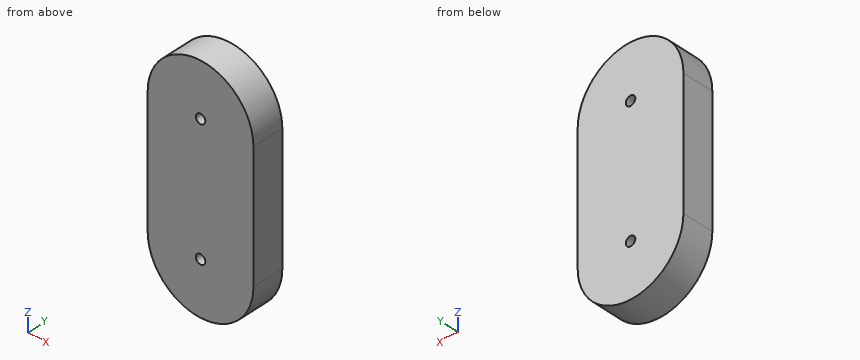
Autodesk Inventor part; units mm, degrees
ref_plane "YZ Plane" through (0, 0, 0) normal (1, 0, 0) x (0, 1, 0)
ref_plane "XZ Plane" through (0, 0, 0) normal (0, 1, 0) x (-1, 0, 0)
ref_plane "XY Plane" through (0, 0, 0) normal (0, 0, 1) x (1, 0, 0)
sketch "Sketch1" plane through (0, 0, 0) normal (0, 1, 0) x (-1, 0, 0)
  line L0 (0, 0) -> (-5.6352, 0)
  line L1 (-5.6352, 0) -> (0, 0)
  line L2 (0, 0) -> (0, 8.7024)
  line L3 (6.5, 14) -> (-6.5, 14)
  line L4 (-6.5, 14) -> (-6.5, 0)
  line L5 (-6.5, 0) -> (6.5, 0)
  line L6 (6.5, 0) -> (6.5, 14)
  circle A0 centre (0, -5) radius 0.9
  circle A1 centre (0, 19) radius 0.9
  line L7 (0, 19) -> (0, -5)
  line L8 (0, 19) -> (0, -5) construction
  line L9 (-10, 19) -> (-10, -5)
  line L10 (10, -5) -> (10, 19)
  arc A2 (10, 19) -> (-10, 19) centre (0, 19) ccw
  arc A3 (-10, -5) -> (10, -5) centre (0, -5) ccw
  point P0 (0, -8.7024)
  point P1 (0, 7)
  dimension "d25" = 13
  dimension "d26" = 14
  dimension "d30" = 5
  dimension "d31" = 5
  dimension "d32" = 1.8
  dimension "d33" = 20
extrude "Extrusion1" add sketch "Sketch1" along normal blind 6 contours L0 L5 L4 L3 L7 L2 | L2 L7 L3 L6 L5 | A2 L10 A3 L9
properties part number "case_usb_cap" material "Acrylic, Clear"
Design review of the part built by this model. Coordinates are the model's own, in mm. Give positions to 0.01 mm unless a question says otherwise; leave off trailing zeros. Order: outer loops, then holes, each group sorted by start corner. A loop starts at its lowest first (then second) coordinate and runs counter-clockwise, first axis right, second up. Notation, with made-up numbers: (51.5, -13) - (74.5, -13) arc R21 ccw to (74.5, -9) - close; hole circle Ø9 at (44.25, 24). An arc over 180 degrees is marked (long way). Use CSV: the item, a comma, the result in double quotes. Start each with the question number.
Q1. Take a section at B-B (y = 0.9). State the section outline as (x, z) points, and give its area (3 significant figures).
Q2. Take a section at D-D (x = -7.5). State the section outline as (y, z) points.
Q3. For P1, Ø3, axis at x = -6, y = 2, coming from the +Z side; P2, Ø1.6, axis at x = 0, z = -5, coming from the -Y side; P3, Ø1.5, axis at x = -3, y = 0.5, coming from the -Z side, all flat-tipped, find the tip position at first contact; note any pin that passes through.
Q4. For line 1 (Z direction, x = 0, y = 3.1); line 2 (X direction, y = 2.7, z = -5); line 3 (Z direction, x = -1.25, y = 0.9), list the stretches that pass through material, from the lowest coordinate up.
Q5. Take a section at C-C (z = -10.5). State the section outline as (x, y) points, and give its area (3 significant figures).
Q6. Take a section at A-A (x = 0). State the section outline as (y, z) points.
Calculated:
1,outline,"(-10, -5) arc R10 ccw to (10, -5) - (10, 19) arc R10 ccw to (-10, 19) - close; hole circle Ø1.8 at (0, -5); hole circle Ø1.8 at (0, 19)"
1,area,"789 mm²"
2,outline,"(0, -11.61) - (6, -11.61) - (6, 25.61) - (0, 25.61) - close"
3,P1,"stops at z = 27.93"
3,P2,"passes through"
3,P3,"stops at z = -14.74"
4,line 1,"z = -15 to -5.9, -4.1 to 18.1, 19.9 to 29"
4,line 2,"x = -10 to -0.9, 0.9 to 10"
4,line 3,"z = -14.92 to 28.92"
5,outline,"(-8.35, 0) - (8.35, 0) - (8.35, 6) - (-8.35, 6) - close"
5,area,"100 mm²"
6,outline,"(0, -15) - (6, -15) - (6, -5.9) - (0, -5.9) - close; (0, -4.1) - (6, -4.1) - (6, 18.1) - (0, 18.1) - close; (0, 19.9) - (6, 19.9) - (6, 29) - (0, 29) - close"
